```python
from build123d import *

# Parameters (mm, degrees)
SKETCH1_W           = 350
SKETCH1_H           = 405
SKETCH1_W_2         = 270
SKETCH1_H_2         = 325
BOSS_EXTRUDE1_DEPTH = 150
SKETCH2_R           = 37.5
CUT_EXTRUDE1_DEPTH  = 40
SKETCH3_R           = 20
CUT_EXTRUDE2_DEPTH  = 40
SKETCH4_R           = 30
CUT_EXTRUDE3_DEPTH  = 40
CHAMFER1_SIZE       = 50
CHAMFER2_SIZE       = 50
CHAMFER3_SIZE       = 50


with BuildPart() as part:
    # Sketch1 → Boss-Extrude1 (new, symmetric)
    with BuildSketch(Plane.XY):
        with Locations((42.392307941, -7.5)):
            Rectangle(SKETCH1_W, SKETCH1_H)
        with Locations((42.392307941, -7.5)):
            Rectangle(SKETCH1_W_2, SKETCH1_H_2, mode=Mode.SUBTRACT)
    extrude(amount=BOSS_EXTRUDE1_DEPTH, both=True)

    # Sketch2 → Cut-Extrude1 (cut)
    with BuildSketch(Plane.ZY.offset(132.607692059)):
        with Locations(Location((0, 0, 0), (0, 0, 270))):
            Circle(SKETCH2_R)
    extrude(amount=-CUT_EXTRUDE1_DEPTH, mode=Mode.SUBTRACT)

    # Sketch3 → Cut-Extrude2 (cut)
    with BuildSketch(Plane(origin=(217.392307941, 0, 0), x_dir=(0, 0, -1), z_dir=(1, 0, 0))):
        with Locations(Location((0, 0, 0), (0, 0, 90))):
            Circle(SKETCH3_R)
    extrude(amount=-CUT_EXTRUDE2_DEPTH, mode=Mode.SUBTRACT)

    # Sketch4 → Cut-Extrude3 (cut)
    with BuildSketch(Plane(origin=(0, 195, 0), x_dir=(1, 0, 0), z_dir=(0, 1, 0))):
        with Locations(Location((53.882307941, 0, 0), (0, 0, 270))):
            Circle(SKETCH4_R)
    extrude(amount=-CUT_EXTRUDE3_DEPTH, mode=Mode.SUBTRACT)

    # Chamfer1
    chamfer1_edges = [part.edges().sort_by_distance(p)[0] for p in [
        (-132.607692059, 195, 0),
        (217.392307941, 195, 0),
        (217.392307941, -210, 0),
        (-132.607692059, -210, 0),
    ]]
    chamfer(chamfer1_edges, length=CHAMFER1_SIZE)

    # Chamfer2
    # the kernel refuses this chamfer: 50 mm, written as the material it takes off along each edge
    with BuildSketch(Plane(origin=(295.97645734, -210, -150), x_dir=(0, 0.9996219169112966, -0.027495876610586587), z_dir=(-1, 0, 0)), Plane(origin=(-211.191841457, 195, 150), x_dir=(0, 0.027495876610586594, -0.9996219169112966), z_dir=(1, 0, 0))) as chamfer2_piece_1:
        Polygon((CHAMFER2_SIZE * 0.999621916911, -CHAMFER2_SIZE * 0.0274958766106), (-CHAMFER2_SIZE * 0.0274958766106, -CHAMFER2_SIZE * 0.999621916911), (0, 0), align=None)
    extrude(amount=507.168298797, mode=Mode.SUBTRACT)
    with BuildSketch(Plane(origin=(-211.191841457, 195, -150), x_dir=(0, 0.027495876610586594, 0.9996219169112966), z_dir=(1, 0, 0)), Plane(origin=(295.97645734, -210, 150), x_dir=(0, 0.9996219169112966, 0.027495876610586587), z_dir=(-1, 0, 0))) as chamfer2_piece_2:
        Polygon((CHAMFER2_SIZE * 0.999621916911, CHAMFER2_SIZE * 0.0274958766106), (-CHAMFER2_SIZE * 0.0274958766106, CHAMFER2_SIZE * 0.999621916911), (0, 0), align=None)
    extrude(amount=507.168298797, mode=Mode.SUBTRACT)

    # Chamfer3
    # the kernel refuses this chamfer: 50 mm, written as the material it takes off along each edge
    with BuildSketch(Plane(origin=(217.392307941, 273.584149398, 150), x_dir=(-0.9996219169112966, 0, 0.027495876610586587), z_dir=(0, -1, 0)), Plane(origin=(-132.607692059, -288.584149398, -150), x_dir=(-0.027495876610586594, 0, 0.9996219169112966), z_dir=(0, 1, 0)), Plane(origin=(217.392307941, 273.584149398, -150), x_dir=(0.027495876610586594, 0, 0.9996219169112966), z_dir=(0, -1, 0))) as chamfer3_piece_1:
        Polygon((CHAMFER3_SIZE * 0.999621916911, CHAMFER3_SIZE * 0.0274958766106), (-CHAMFER3_SIZE * 0.0274958766106, CHAMFER3_SIZE * 0.999621916911), (0, 0), align=None)
    extrude(amount=562.168298797, mode=Mode.SUBTRACT)
    with BuildSketch(Plane(origin=(-132.607692059, -288.584149398, 150), x_dir=(-0.027495876610586594, 0, -0.9996219169112966), z_dir=(0, 1, 0))) as chamfer3_piece_2:
        Polygon((CHAMFER3_SIZE * 0.999621916911, -CHAMFER3_SIZE * 0.0274958766106), (-CHAMFER3_SIZE * 0.0274958766106, -CHAMFER3_SIZE * 0.999621916911), (0, 0), align=None)
    extrude(amount=562.168298797, mode=Mode.SUBTRACT)


solid = part.part
```
Input: part model. Units: mm. Frame: model coordinates. A direction names the side the tool comes from. Give positions to 0.01 mm unless a question says otherwise; leave off trailing zeros. Order: outer loops, then holes, each group sorted by start corner. A loop starts at its lowest first (then second) coordinate and runs counter-clockwise, first axis right, second up. Notation, with made-up numbers: (53.25, 69) - (103.25, 69) arc R12 ccw to (103.25, 75) - close; hole circle Ø3 at (27, -3). An arc over 180 degrees is marked (long way). Use a Markdown table: item, result.
(1) Pin query (flat end, axial travel): pin 1 (6 mm diameter, centred on x = -92.5, z = -82, fed in from +Y); pin 2 (1 mm diameter, centred on x = -88.5, z = -103.5, fed in from -Y). Return the tip coordinate at first contact, or that it passes through.
Computed values:
| item | result |
|---|---|
| pin 1 | stops at y = 188.11 |
| pin 2 | stops at y = -204.61 |
(2) Section query C-C (y = -84.5). Output: boundary loops of the cut face in (x, z).
Computed values:
| item | result |
|---|---|
| outline | (-132.61, -100) - (-92.61, -140) - (-92.61, 140) - (-132.61, 100) - close; (177.39, -140) - (217.39, -100) - (217.39, 100) - (177.39, 140) - close |
(3) Draft query along X for faces 1 (the cylindrical face through (-112.888, 29.759, -22.818)), 2 (the flat face through (11, 155, 2)), 3 (the flat face through (192.74, 169.65, 1.75)), 4 (the flat face through (177.392, -10, 33)). Return one class per face: released by +X, released by -X, zero draft, split by the parting line, or undercut.
Computed values:
| item | result |
|---|---|
| face 1 | zero draft |
| face 2 | undercut |
| face 3 | released by +X |
| face 4 | undercut |
(4) Section query A-A (x = 130.5). Output: boundary loops of the cut face in (y, z).
Computed values:
| item | result |
|---|---|
| outline | (-210, -100) - (-170, -140) - (-170, 140) - (-210, 100) - close; (155, -140) - (195, -100) - (195, 100) - (155, 140) - close |
(5) Access query for faces 5 (the cylindrical face through (83.627, 175.28, -3.905)), 6 (the flat face through (41, -170, 2)), 7 (the flat face through (197.67, -5.01, -119.72)). Directions: +Z, -Z, +X, -X, +Y, -Y. A direction counts if a zero-diameter tool reaches every point of the face in a straight line with its end or side. Return the directions, or none.
Computed values:
| item | result |
|---|---|
| face 5 | +Y |
| face 6 | +Z, -Z |
| face 7 | -Z, +X, +Y, -Y |
(6) Section query B-B (z = 0). Output: boundary loops of the cut face in (x, y), then the cut area to 3 significant figures.
Computed values:
| item | result |
|---|---|
| outline | (-132.61, -160) - (-82.61, -210) - (167.39, -210) - (217.39, -160) - (217.39, -20) - (177.39, -20) - (177.39, -170) - (-92.61, -170) - (-92.61, -37.5) - (-132.61, -37.5) - close; (-132.61, 37.5) - (-92.61, 37.5) - (-92.61, 155) - (23.88, 155) - (23.88, 195) - (-82.61, 195) - (-132.61, 145) - close; (83.88, 155) - (177.39, 155) - (177.39, 20) - (217.39, 20) - (217.39, 145) - (167.39, 195) - (83.88, 195) - close |
| area | 42,000 mm2 |
(7) Section query D-D (y = 0). Output: boundary loops of the cut face in (x, z).
Computed values:
| item | result |
|---|---|
| outline | (-132.61, -100) - (-92.61, -140) - (-92.61, -37.5) - (-132.61, -37.5) - close; (-132.61, 37.5) - (-92.61, 37.5) - (-92.61, 140) - (-132.61, 100) - close; (177.39, -140) - (217.39, -100) - (217.39, -20) - (177.39, -20) - close; (177.39, 20) - (217.39, 20) - (217.39, 100) - (177.39, 140) - close |
(8) Line query: line 1 (X direction, y = 107, z = 28); line 2 (Y direction, x = -10.5, z = -74); line 3 (X direction, y = -139, z = 121.5). Output: solid intervals per line, ascending. Write a range as from..to.
Computed values:
| item | result |
|---|---|
| line 1 | x = -132.61..-92.61, 177.39..217.39 |
| line 2 | y = -210..-170, 155..195 |
| line 3 | x = -111.11..-92.61, 177.39..195.89 |
